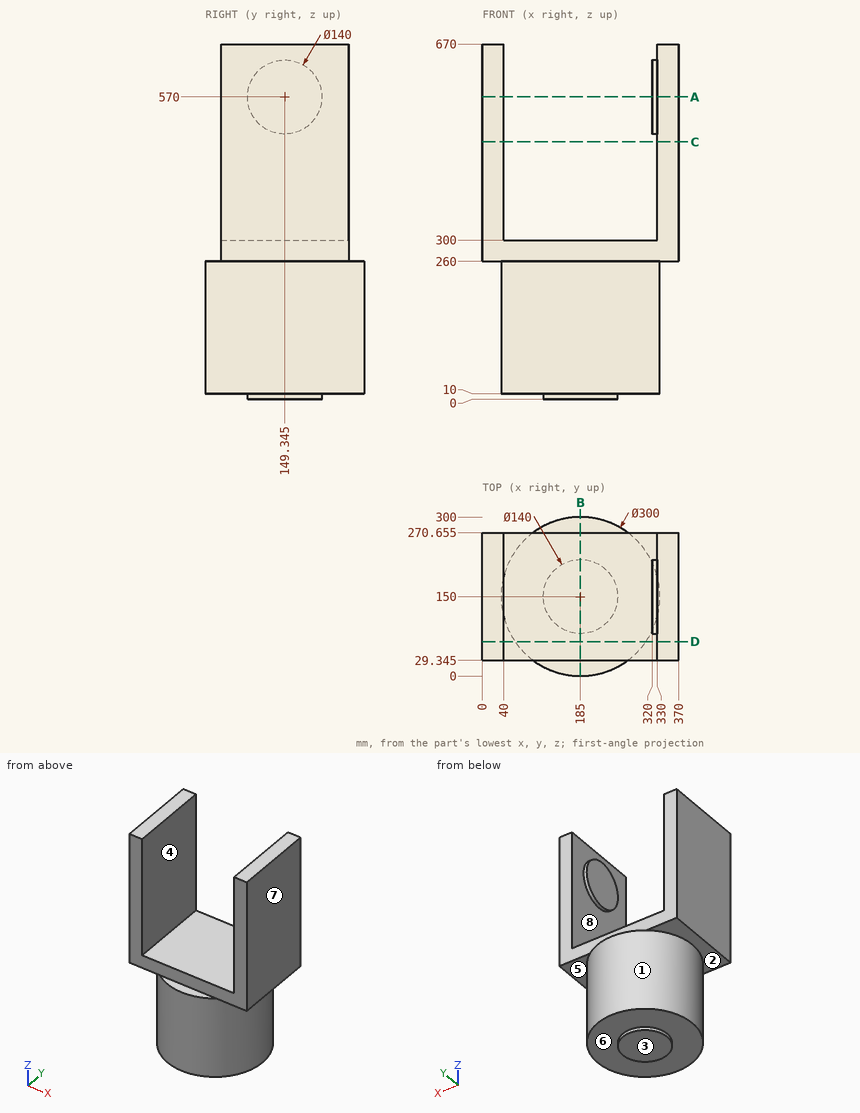
Print and shaded views of the part. All mm, measured from the part's lowest x, y and z. A direction names the side the tool comes from. Coordinates: 2 decimals unless noted, no trailing zeros. Write each loop counter-clockwise with the first axis right and the second up, starting at its lowest first coordinate (ties: lowest second). Pieces come first, ordered by that corner, then holes.
(1) Two-plate mould, pull along Z, no slides. Class the marked faces 6, 7 and 8: +Z half, -Z half, draft (parallel to the pull), parting line (faces both ways), or undercut.
(2) Cut at C-C, the plane z = 485.5. List the corners of the cut face in (x, y) (1 decimal), and give its area (3 significant figures).
(3) 3-axis set-ups, long thin cutter, end or side, ignore diameter. For the marked faces 1, 2, 3, 4 and 5: which of +Z, -Z, +X, -X, +Y, -Y reach the whole face in a straight line?
(4) Drill centre lines: probe 1 along X at (y, z) = (40, 352); probe 2 along X at (y, z) = (143, 548.5); probe 3 along Z at (x, y) = (288.5, 164). Where is each one in solid material? Low to high.
(5) Cut at A-A, the plane z = 570. List the corners of the cut face in (x, y) (1 decimal).
(6) Cut at B-B, the plane x = 185. List the corners of the cut face in (y, z) (1 decimal).
(7) Cut at D-D, the plane y = 65. List the corners of the cut face in (x, z), and give its area (3 significant figures).
(8) Flat gauge pins, fed straight in: pin 1 (4 mm diameter, centred on x = 251, z = 269, fed in from -Y) (1 decimal); pin 2 (23.5 mm diameter, centred on x = 202.5, y = 16, fed in from +Z); pin 3 (4 mm diameter, centred on x = 115.5, y = 226, fed in from -Z). Where does each tip first touch, or does it go through?
Geometry says:
1. face 6: -Z half
1. face 7: draft
1. face 8: undercut
2. outline: (0, 29.3) - (40, 29.3) - (40, 270.7) - (0, 270.7) - close; (330, 29.3) - (370, 29.3) - (370, 270.7) - (330, 270.7) - close
2. area: 19,300 mm2
3. face 1: -Z
3. face 2: -Z, -X
3. face 3: -Z, +X, -X, +Y, -Y
3. face 4: +Z, +Y, -Y
3. face 5: -Z, +X
4. probe 1: x = 0 to 40, 330 to 370
4. probe 2: x = 0 to 40, 320 to 370
4. probe 3: z = 10 to 300
5. outline: (0, 29.3) - (40, 29.3) - (40, 270.7) - (0, 270.7) - close; (320, 79.3) - (330, 79.3) - (330, 29.3) - (370, 29.3) - (370, 270.7) - (330, 270.7) - (330, 219.3) - (320, 219.3) - close
6. outline: (0, 10) - (80, 10) - (80, 0) - (220, 0) - (220, 10) - (300, 10) - (300, 260) - (270.7, 260) - (270.7, 300) - (29.3, 300) - (29.3, 260) - (0, 260) - close
7. outline: (0, 260) - (61.41, 260) - (61.41, 10) - (308.59, 10) - (308.59, 260) - (370, 260) - (370, 670) - (330, 670) - (330, 300) - (40, 300) - (40, 670) - (0, 670) - close
7. area: 106,000 mm2
8. pin 1: stops at y = 29.3
8. pin 2: stops at z = 260
8. pin 3: stops at z = 10
